```python
from build123d import *

# Parameters (mm, degrees)
SKETCH_1_W      = 710
SKETCH_1_H      = 10
SKETCH_1_R      = 1.6
EXTRUDE_1_DEPTH = 7


with BuildPart() as part:
    # 草图1 → 凸台-拉伸1 (new body)
    with BuildSketch(Plane(origin=(0, 0, 0), x_dir=(1, 0, 0), z_dir=(0, 1, 0))):
        Rectangle(SKETCH_1_W, SKETCH_1_H)
        with Locations(Location((-345, 0, 0), (0, 0, 270))):
            Circle(SKETCH_1_R, mode=Mode.SUBTRACT)
        with Locations(Location((-325, 0, 0), (0, 0, 270))):
            Circle(SKETCH_1_R, mode=Mode.SUBTRACT)
        with Locations(Location((-305, 0, 0), (0, 0, 270))):
            Circle(SKETCH_1_R, mode=Mode.SUBTRACT)
        with Locations(Location((-285, 0, 0), (0, 0, 270))):
            Circle(SKETCH_1_R, mode=Mode.SUBTRACT)
        with Locations(Location((-265, 0, 0), (0, 0, 270))):
            Circle(SKETCH_1_R, mode=Mode.SUBTRACT)
        with Locations(Location((-245, 0, 0), (0, 0, 270))):
            Circle(SKETCH_1_R, mode=Mode.SUBTRACT)
        with Locations(Location((-225, 0, 0), (0, 0, 270))):
            Circle(SKETCH_1_R, mode=Mode.SUBTRACT)
        with Locations(Location((-205, 0, 0), (0, 0, 270))):
            Circle(SKETCH_1_R, mode=Mode.SUBTRACT)
        with Locations(Location((-185, 0, 0), (0, 0, 270))):
            Circle(SKETCH_1_R, mode=Mode.SUBTRACT)
        with Locations(Location((-165, 0, 0), (0, 0, 270))):
            Circle(SKETCH_1_R, mode=Mode.SUBTRACT)
        with Locations(Location((-145, 0, 0), (0, 0, 270))):
            Circle(SKETCH_1_R, mode=Mode.SUBTRACT)
        with Locations(Location((-125, 0, 0), (0, 0, 270))):
            Circle(SKETCH_1_R, mode=Mode.SUBTRACT)
        with Locations(Location((-105, 0, 0), (0, 0, 270))):
            Circle(SKETCH_1_R, mode=Mode.SUBTRACT)
        with Locations(Location((-85, 0, 0), (0, 0, 270))):
            Circle(SKETCH_1_R, mode=Mode.SUBTRACT)
        with Locations(Location((-65, 0, 0), (0, 0, 270))):
            Circle(SKETCH_1_R, mode=Mode.SUBTRACT)
        with Locations(Location((-45, 0, 0), (0, 0, 270))):
            Circle(SKETCH_1_R, mode=Mode.SUBTRACT)
        with Locations(Location((-25, 0, 0), (0, 0, 270))):
            Circle(SKETCH_1_R, mode=Mode.SUBTRACT)
        with Locations(Location((-5, 0, 0), (0, 0, 270))):
            Circle(SKETCH_1_R, mode=Mode.SUBTRACT)
        with Locations(Location((15, 0, 0), (0, 0, 270))):
            Circle(SKETCH_1_R, mode=Mode.SUBTRACT)
        with Locations(Location((35, 0, 0), (0, 0, 270))):
            Circle(SKETCH_1_R, mode=Mode.SUBTRACT)
        with Locations(Location((55, 0, 0), (0, 0, 270))):
            Circle(SKETCH_1_R, mode=Mode.SUBTRACT)
        with Locations(Location((75, 0, 0), (0, 0, 270))):
            Circle(SKETCH_1_R, mode=Mode.SUBTRACT)
        with Locations(Location((95, 0, 0), (0, 0, 270))):
            Circle(SKETCH_1_R, mode=Mode.SUBTRACT)
        with Locations(Location((115, 0, 0), (0, 0, 270))):
            Circle(SKETCH_1_R, mode=Mode.SUBTRACT)
        with Locations(Location((135, 0, 0), (0, 0, 270))):
            Circle(SKETCH_1_R, mode=Mode.SUBTRACT)
        with Locations(Location((155, 0, 0), (0, 0, 270))):
            Circle(SKETCH_1_R, mode=Mode.SUBTRACT)
        with Locations(Location((175, 0, 0), (0, 0, 270))):
            Circle(SKETCH_1_R, mode=Mode.SUBTRACT)
        with Locations(Location((195, 0, 0), (0, 0, 270))):
            Circle(SKETCH_1_R, mode=Mode.SUBTRACT)
        with Locations(Location((215, 0, 0), (0, 0, 270))):
            Circle(SKETCH_1_R, mode=Mode.SUBTRACT)
        with Locations(Location((235, 0, 0), (0, 0, 270))):
            Circle(SKETCH_1_R, mode=Mode.SUBTRACT)
        with Locations(Location((255, 0, 0), (0, 0, 270))):
            Circle(SKETCH_1_R, mode=Mode.SUBTRACT)
        with Locations(Location((275, 0, 0), (0, 0, 270))):
            Circle(SKETCH_1_R, mode=Mode.SUBTRACT)
        with Locations(Location((295, 0, 0), (0, 0, 270))):
            Circle(SKETCH_1_R, mode=Mode.SUBTRACT)
        with Locations(Location((315, 0, 0), (0, 0, 270))):
            Circle(SKETCH_1_R, mode=Mode.SUBTRACT)
        with Locations(Location((335, 0, 0), (0, 0, 270))):
            Circle(SKETCH_1_R, mode=Mode.SUBTRACT)
    extrude(amount=EXTRUDE_1_DEPTH)


solid = part.part
```
Geometry: final body of the model. Coordinates: model frame, mm. Give positions to 0.01 mm unless a question says otherwise; leave off trailing zeros. Use CSV: the item, a comma, the result in double quotes.
(1) Ray query, line 1 along Z through (x, y) = (115, 2.25). Return the intervals inside material, ascending. Write a range as [from, to].
From the geometry:
line 1,"[-5, -1.6], [1.6, 5]"
(2) Cut plane A-A (y = 2). Count the separate pieces of the cut face and the enclosed holes in it, plus the area to 3 significant figures.
From the geometry:
separate pieces,"1"
enclosed holes,"35"
area,"6,820 mm^2"
(3) First-contact query: P1, Ø3.5, axis at x = -165, z = 0, coming from the +Y side. Flat tip, straight axial feed; report the tip coordinate or a pass-through.
From the geometry:
P1,"y = 7"
